from build123d import *

# Parameters (mm, degrees)
BOSS_EXTRUDE1_DEPTH    = 5
BOSS_EXTRUDE2_START    = 8
SKETCH2_R              = 4
BOSS_EXTRUDE2_DEPTH    = 8
CUT_EXTRUDE1_DEPTH     = 8
SKETCH4_R              = 1.25
CUT_EXTRUDE2_DEPTH     = 8
CUT_EXTRUDE3_START     = -2.5
CUT_EXTRUDE3_OUTLINE_R = 1.25
CUT_EXTRUDE3_DEPTH     = 2.5


# Read off the part's stored shape, not the designer's step: Cut-Extrude3
with BuildPart() as part:
    # Sketch1 → Boss-Extrude1 (new body)
    with BuildSketch(Plane.XY):
        with BuildLine():
            Line((-1.936491673, 3.5), (1.936491673, 3.5))
            ThreePointArc((1.936491673, 3.5), (0, -4), (-1.936491673, 3.5))
        make_face()
    extrude(amount=BOSS_EXTRUDE1_DEPTH)

    # Sketch2 → Boss-Extrude2 (add)
    with BuildSketch(Plane(origin=(0, 0, 0), x_dir=(-1, 0, 0), z_dir=(0, 0, -1)).offset(BOSS_EXTRUDE2_START)):
        Circle(SKETCH2_R)
    extrude(amount=-BOSS_EXTRUDE2_DEPTH)

    # Sketch3 → Cut-Extrude1 (cut)
    with BuildSketch(Plane(origin=(0, 0, -8), x_dir=(-1, 0, 0), z_dir=(0, 0, -1))):
        with BuildLine():
            Line((-1.322875656, 1.5), (1.322875656, 1.5))
            ThreePointArc((1.322875656, 1.5), (0, -2), (-1.322875656, 1.5))
        make_face()
    extrude(amount=-CUT_EXTRUDE1_DEPTH, mode=Mode.SUBTRACT)

    # Sketch4 → Cut-Extrude2 (cut)
    with BuildSketch(Plane.XY.offset(5)):
        Circle(SKETCH4_R)
    extrude(amount=-CUT_EXTRUDE2_DEPTH, mode=Mode.SUBTRACT)

    # Cut-Extrude3 outline → Cut-Extrude3 (cut)
    with BuildSketch(Plane(origin=(0, 4, 0), x_dir=(1, 0, 0), z_dir=(0, 1, 0)).offset(CUT_EXTRUDE3_START)):
        with Locations((0, 4)):
            Circle(CUT_EXTRUDE3_OUTLINE_R)
    extrude(amount=CUT_EXTRUDE3_DEPTH, mode=Mode.SUBTRACT)


solid = part.part
Verification items for the finished model (mm, model axes). A direction names the side the tool comes from. Give positions to 0.01 mm unless a question says otherwise; leave off trailing zeros. Loops run counter-clockwise (first coordinate to the right, second up) from the corner with the lowest first, then second, coordinate; pieces in that order, holes last. Notation, with made-up numbers: (-29.75, -9.5) - (23.25, -9.5) arc R15 ccw to (23.25, 11.5) - close; hole circle Ø1 at (7, -28.5). An arc over 180 degrees is marked (long way). Write each question's results on one line, items separated by ' | '.
1) Sectioned sample at B-B on y = -0.25. Record the boundary of the cut face in (x, z).
Solution:
outline: (-3.99, -8) - (-1.98, -8) - (-1.98, 0) - (-1.22, 0) - (-1.22, 5) - (-3.99, 5) - close; (1.22, 0) - (1.98, 0) - (1.98, -8) - (3.99, -8) - (3.99, 5) - (1.22, 5) - close
2) Material ranges on L1, parallel to Y at x = 0, z = -5.75; L2, parallel to Z at x = 0, y = 3.45; L3, parallel to Y at x = 0, z = 2, recorded low to high. Write a range as from..to.
Solution:
L1: -4..-2, 1.5..4 | L2: -8..-5.25, -2.75..5 | L3: -4..-1.25, 1.25..3.5
3) Sectioned sample at D-D on x = -1.5. Record the boundary of the cut face in (y, z), plus the area to 3 significant figures.
Solution:
outline: (-3.71, -8) - (-1.32, -8) - (-1.32, 0) - (1.32, 0) - (1.32, -8) - (3.71, -8) - (3.71, 0) - (3.5, 0) - (3.5, 5) - (-3.71, 5) - close | area: 74.2 mm2
4) Sectioned sample at C-C on z = -6. Record the boundary of the cut face in (x, y).
Solution:
outline: circle Ø8 at (0, 0); hole (-1.32, 1.5) arc R2 ccw (long way) to (1.32, 1.5) - close
5) Depth check by flat-ended pin: P1, Ø1.2, axis at x = -0.5, z = 3.5, coming from the +Y side. Enter the tip coordinate at first touch or a pass-through.
Solution:
P1: y = 3.5
6) Sectioned sample at A-A on x = 0.25. Record the boundary of the cut face in (y, z), plus the area to 3 significant figures.
Solution:
outline: (-3.99, -8) - (-1.98, -8) - (-1.98, 0) - (-1.22, 0) - (-1.22, 5) - (-3.99, 5) - close; (1.22, 0) - (1.5, 0) - (1.5, -2.78) - (3.99, -2.78) - (3.99, 0) - (3.5, 0) - (3.5, 5) - (1.22, 5) - close; (1.5, -8) - (3.99, -8) - (3.99, -5.22) - (1.5, -5.22) - close | area: 55.1 mm2
7) Mould release check, pull along Y, two halves, no side actions. Record for faces 4 (the flat face through (0, 3.5, 2)), 5 (the flat face through (-1, -1, 5)), 6 (the flat face through (1, -1, 0)): pulls with the +Y half, pulls with the -Y half, needs draft (parallel to the pull), parting line crosses it, or undercut.
Solution:
face 4: pulls with the +Y half | face 5: needs draft | face 6: undercut
8) Tool access check on faces 1 (the flat face through (1, 1.5, -5)), 2 (the cylindrical face through (-1.25, 2.73, -4.05)), 3 (the flat face through (0, 2, -8)). Record the directions out of +Z, -Z, +X, -X, +Y, -Y that give a thin tool (end or side, any length) a straight path to the whole face; none if there is none.
Solution:
face 1: -Z | face 2: +Y | face 3: -Z, +X, -X, +Y, -Y
